Check sheet for the modelled part. Datum: model origin and axes. Units: mm. Coordinates: 2 decimals unless noted, no trailing zeros. Loops run counter-clockwise (first coordinate to the right, second up) from the corner with the lowest first, then second, coordinate; pieces in that order, holes last.
```python
from build123d import *

# Parameters (mm, degrees)
AXLE_SUPPORT_PLATE_R   = 7.030128061
AXLE_SUPPORT_PLATE_R_2 = 2.159
AXLE_SUPPORT_PLATE_W   = 6.35
AXLE_SUPPORT_PLATE_H   = 6.35
BOSS_EXTRUDE1_DEPTH    = 6.35


with BuildPart() as part:
    # Axle Support Plate → Boss-Extrude1 (new body)
    with BuildSketch(Plane(origin=(0, 0, 0), x_dir=(1, 0, 0), z_dir=(0, 1, 0))):
        Polygon((63.58606403, -169.56756403), (63.58606403, -1.972692091), (145.546192091, -1.972692091), (145.546192091, 8.23243597), (158.246192091, 8.23243597), (158.246192091, 14.58243597), (145.546192091, 14.58243597), (145.546192091, 24.78756403), (63.58606403, 24.78756403), (63.58606403, 169.56756403), (-63.58606403, 169.56756403), (-63.58606403, 63.35043597), (-69.93606403, 63.35043597), (-69.93606403, 57.00043597), (-63.58606403, 57.00043597), (-63.58606403, 50.65043597), (-58.051064051, 50.65043597), (-58.051064051, 52.691435952), (-55.151064009, 52.691435952), (-55.151064009, 50.65043597), (-49.61606403, 50.65043597), (-49.61606403, 46.33243597), (-55.151064009, 46.33243597), (-55.151064009, 44.291435988), (-58.051064051, 44.291435988), (-58.051064051, 46.33243597), (-63.58606403, 46.33243597), (-63.58606403, 39.98243597), (-69.93606403, 39.98243597), (-69.93606403, 33.63243597), (-63.58606403, 33.63243597), (-63.58606403, -63.64956403), (-69.93606403, -63.64956403), (-69.93606403, -69.99956403), (-63.58606403, -69.99956403), (-63.58606403, -76.34956403), (-58.051064051, -76.34956403), (-58.051064051, -74.308564048), (-55.151064009, -74.308564048), (-55.151064009, -76.34956403), (-49.61606403, -76.34956403), (-49.61606403, -80.66756403), (-55.151064009, -80.66756403), (-55.151064009, -82.708564012), (-58.051064051, -82.708564012), (-58.051064051, -80.66756403), (-63.58606403, -80.66756403), (-63.58606403, -87.01756403), (-69.93606403, -87.01756403), (-69.93606403, -93.36756403), (-63.58606403, -93.36756403), (-63.58606403, -169.56756403), (26.07593597, -169.56756403), (26.07593597, -175.91756403), (32.42593597, -175.91756403), (32.42593597, -169.56756403), (38.77593597, -169.56756403), (38.77593597, -164.032564051), (36.734935988, -164.032564051), (36.734935988, -161.132564009), (38.77593597, -161.132564009), (38.77593597, -155.59756403), (43.09393597, -155.59756403), (43.09393597, -161.132564009), (45.134935952, -161.132564009), (45.134935952, -164.032564051), (43.09393597, -164.032564051), (43.09393597, -169.56756403), (49.44393597, -169.56756403), (49.44393597, -175.91756403), (55.79393597, -175.91756403), (55.79393597, -169.56756403), align=None)
        with Locations(Location((51.47593597, 157.45743597, 0), (0, 0, 270))):
            Circle(AXLE_SUPPORT_PLATE_R, mode=Mode.SUBTRACT)
        with Locations(Location((51.47593597, -134.64256403, 0), (0, 0, 270))):
            Circle(AXLE_SUPPORT_PLATE_R, mode=Mode.SUBTRACT)
        with Locations(Location((41.95093597, 89.76643597, 0), (0, 0, 270))):
            Circle(AXLE_SUPPORT_PLATE_R_2, mode=Mode.SUBTRACT)
        with Locations(Location((41.95093597, -66.95156403, 0), (0, 0, 270))):
            Circle(AXLE_SUPPORT_PLATE_R_2, mode=Mode.SUBTRACT)
        Polygon((0, 156.86756403), (-15.875, 140.99256403), (-3.175, 140.99256403), (-15.875, 128.29256403), (-3.175, 128.29256403), (-15.875, 115.59256403), (-3.175, 115.59256403), (-15.875, 102.89256403), (-3.175, 102.89256403), (-15.875, 90.19256403), (-3.175, 90.19256403), (-15.875, 77.49256403), (-3.175, 77.49256403), (-15.875, 64.79256403), (-3.175, 64.79256403), (-15.875, 52.09256403), (-3.175, 52.09256403), (-15.875, 39.39256403), (-3.175, 39.39256403), (-15.875, 26.69256403), (-3.175, 26.69256403), (-15.875, 13.99256403), (-3.175, 13.99256403), (-15.875, 1.29256403), (-3.175, 1.29256403), (-15.875, -11.40743597), (-3.175, -11.40743597), (-15.875, -24.10743597), (-3.175, -24.10743597), (-15.875, -36.80743597), (-3.175, -36.80743597), (-15.875, -49.50743597), (-3.175, -49.50743597), (-15.875, -62.20743597), (-3.175, -62.20743597), (-15.875, -74.90743597), (-3.175, -74.90743597), (-15.875, -87.60743597), (-3.175, -87.60743597), (-15.875, -100.30743597), (-3.175, -100.30743597), (-15.875, -113.00743597), (-3.175, -113.00743597), (-15.875, -125.70743597), (-3.175, -125.70743597), (-15.875, -138.40743597), (-3.175, -138.40743597), (-15.875, -151.10743597), (15.875, -151.10743597), (3.175, -138.40743597), (15.875, -138.40743597), (3.175, -125.70743597), (15.875, -125.70743597), (3.175, -113.00743597), (15.875, -113.00743597), (3.175, -100.30743597), (15.875, -100.30743597), (3.175, -87.60743597), (15.875, -87.60743597), (3.175, -74.90743597), (15.875, -74.90743597), (3.175, -62.20743597), (15.875, -62.20743597), (3.175, -49.50743597), (15.875, -49.50743597), (3.175, -36.80743597), (15.875, -36.80743597), (3.175, -24.10743597), (15.875, -24.10743597), (3.175, -11.40743597), (15.875, -11.40743597), (3.175, 1.29256403), (15.875, 1.29256403), (3.175, 13.99256403), (15.875, 13.99256403), (3.175, 26.69256403), (15.875, 26.69256403), (3.175, 39.39256403), (15.875, 39.39256403), (3.175, 52.09256403), (15.875, 52.09256403), (3.175, 64.79256403), (15.875, 64.79256403), (3.175, 77.49256403), (15.875, 77.49256403), (3.175, 90.19256403), (15.875, 90.19256403), (3.175, 102.89256403), (15.875, 102.89256403), (3.175, 115.59256403), (15.875, 115.59256403), (3.175, 128.29256403), (15.875, 128.29256403), (3.175, 140.99256403), (15.875, 140.99256403), align=None, mode=Mode.SUBTRACT)
        with BuildLine():
            Line((70.616192091, 18.43756403), (108.716192091, 18.43756403))
            ThreePointArc((108.716192091, 18.43756403), (115.746320151, 11.40743597), (108.716192091, 4.377307909))
            Line((108.716192091, 4.377307909), (70.616192091, 4.377307909))
            ThreePointArc((70.616192091, 4.377307909), (63.58606403, 11.40743597), (70.616192091, 18.43756403))
        make_face(mode=Mode.SUBTRACT)
        with Locations((41.95093597, 101.45043597)):
            Rectangle(AXLE_SUPPORT_PLATE_W, AXLE_SUPPORT_PLATE_H, mode=Mode.SUBTRACT)
        with Locations((41.95093597, 78.08243597)):
            Rectangle(AXLE_SUPPORT_PLATE_W, AXLE_SUPPORT_PLATE_H, mode=Mode.SUBTRACT)
        with Locations((41.95093597, -78.63556403)):
            Rectangle(AXLE_SUPPORT_PLATE_W, AXLE_SUPPORT_PLATE_H, mode=Mode.SUBTRACT)
        with Locations((41.95093597, -55.26756403)):
            Rectangle(AXLE_SUPPORT_PLATE_W, AXLE_SUPPORT_PLATE_H, mode=Mode.SUBTRACT)
    extrude(amount=BOSS_EXTRUDE1_DEPTH)


solid = part.part
```
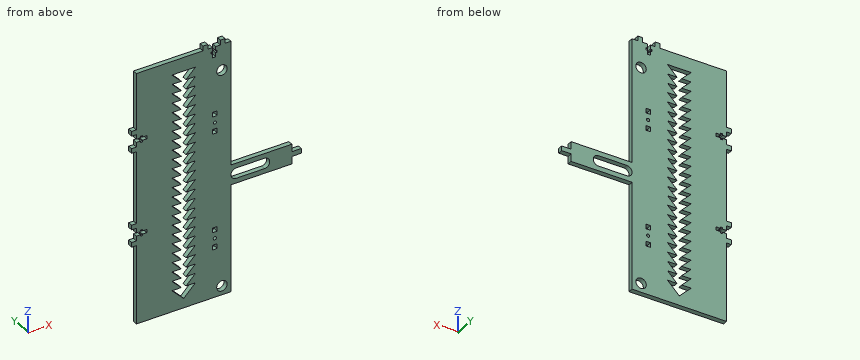
1) Depth check by flat-ended pin: pin 1 (1.5 mm diameter, centred on y = 2, z = 162.5, fed in from +X); pin 2 (1 mm diameter, centred on y = 2, z = 75.5, fed in from -X); pin 3 (1 mm diameter, centred on x = 89.5, y = 2, fed in from -Z). Enter the tip coordinate at first touch or a pass-through.
Answer sheet:
pin 1: stops at x = 63.59
pin 2: stops at x = -63.59
pin 3: stops at z = -24.79
2) Scan lines: line 1 (Z direction, x = -51.5, y = 2.75); line 2 (X direction, y = 4, z = -81); line 3 (Z direction, x = 37, y = 5.5). Record each from-to range of solid material in increasing order.
Answer sheet:
line 1: z = -169.57 to -50.65, -46.33 to 76.35, 80.67 to 169.57
line 2: x = -63.59 to -12.37, 12.37 to 38.78, 45.13 to 63.59
line 3: z = -169.57 to 161.13, 164.03 to 169.57
3) Section check C-C on x = 136.5. Enter the section's corners in (y, z).
Answer sheet:
outline: (0, -24.79) - (6.35, -24.79) - (6.35, 1.97) - (0, 1.97) - close
4) Section check A-A on x = 102.5. Enter the section's corners in (y, z), plus the area to 3 significant figures.
Answer sheet:
outline: (0, -24.79) - (6.35, -24.79) - (6.35, -18.44) - (0, -18.44) - close; (0, -4.38) - (6.35, -4.38) - (6.35, 1.97) - (0, 1.97) - close
area: 80.6 mm2
5) Section check D-D on y = 3. Give the number of separate pieces and of enclosed holes in the cut face, plus the area to 3 significant figures.
Answer sheet:
separate pieces: 1
enclosed holes: 10
area: 38,400 mm2
6) Section check B-B on z = 118.5. Enter the section's corners in (x, y).
Answer sheet:
outline: (-63.59, 0) - (-8.67, 0) - (-8.67, 6.35) - (-63.59, 6.35) - close; (8.67, 0) - (63.59, 0) - (63.59, 6.35) - (8.67, 6.35) - close
